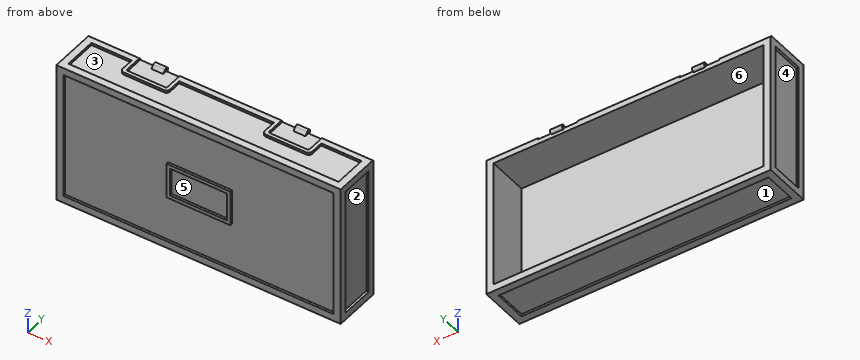
from build123d import *

# Parameters (mm, degrees)
SKETCH1_W                = 120
SKETCH1_H                = 60
BOSS_EXTRUDE1_DEPTH      = 20
SKETCH2_W                = 114
SKETCH2_H                = 54
CUT_EXTRUDE1_DEPTH       = 17
CUT_EXTRUDE2_DEPTH       = 1
CUT_EXTRUDE3_DEPTH       = 1
SKETCH5_W                = 54
SKETCH5_H                = 14
CUT_EXTRUDE4_DEPTH       = 1
SKETCH6_W                = 54
SKETCH6_H                = 14
CUT_EXTRUDE5_DEPTH       = 1
SKETCH7_W                = 114
SKETCH7_H                = 14
CUT_EXTRUDE6_DEPTH       = 1
SKETCH8_W                = 114
SKETCH8_H                = 54
CUT_EXTRUDE7_DEPTH       = 1
BOSS_EXTRUDE2_DEPTH      = 3
BOSS_EXTRUDE2_DEPTH_BACK = 0.5
CUT_EXTRUDE8_DEPTH       = 5
BOSS_EXTRUDE3_DEPTH      = 2
BOSS_EXTRUDE3_DEPTH_BACK = 0.5
CUT_EXTRUDE9_DEPTH       = 5
CUT_EXTRUDE10_DEPTH      = 23
CUT_EXTRUDE11_DEPTH      = 43
CUT_EXTRUDE12_DEPTH      = 43
BOSS_EXTRUDE5_DEPTH      = 1


with BuildPart() as part:
    # Sketch1 → Boss-Extrude1 (new body)
    with BuildSketch(Plane(origin=(0, 0, 0), x_dir=(1, 0, 0), z_dir=(0, 1, 0))):
        with Locations((60, 30)):
            Rectangle(SKETCH1_W, SKETCH1_H)
    extrude(amount=BOSS_EXTRUDE1_DEPTH)

    # Sketch2 → Cut-Extrude1 (cut)
    with BuildSketch(Plane(origin=(0, 20, 0), x_dir=(1, 0, 0), z_dir=(0, 1, 0))):
        with Locations((60, 30)):
            Rectangle(SKETCH2_W, SKETCH2_H)
    extrude(amount=-CUT_EXTRUDE1_DEPTH, mode=Mode.SUBTRACT)

    # Sketch3 → Cut-Extrude2 (cut)
    with BuildSketch(Plane.XY):
        with BuildLine():
            Line((38.5, 20), (21.5, 20))
            Line((21.5, 20), (21.5, 12))
            ThreePointArc((21.5, 12), (21.646446609, 11.646446609), (22, 11.5))
            Line((22, 11.5), (38, 11.5))
            ThreePointArc((38, 11.5), (38.353553391, 11.646446609), (38.5, 12))
            Line((38.5, 12), (38.5, 20))
        make_face()
        with BuildLine():
            Line((98.5, 12), (98.5, 20))
            Line((98.5, 20), (81.5, 20))
            Line((81.5, 20), (81.5, 12))
            ThreePointArc((81.5, 12), (81.646446609, 11.646446609), (82, 11.5))
            Line((82, 11.5), (98, 11.5))
            ThreePointArc((98, 11.5), (98.353553391, 11.646446609), (98.5, 12))
        make_face()
    extrude(amount=-CUT_EXTRUDE2_DEPTH, mode=Mode.SUBTRACT)

    # Sketch4 → Cut-Extrude3 (cut)
    with BuildSketch(Plane.XY):
        with BuildLine():
            Line((20, 17), (3, 17))
            Line((3, 17), (3, 3))
            Line((3, 3), (117, 3))
            Line((117, 3), (117, 17))
            Line((117, 17), (100, 17))
            Line((100, 17), (100, 11.5))
            ThreePointArc((100, 11.5), (99.560660172, 10.439339828), (98.5, 10))
            Line((98.5, 10), (81.5, 10))
            ThreePointArc((81.5, 10), (80.439339828, 10.439339828), (80, 11.5))
            Line((80, 11.5), (80, 17))
            Line((80, 17), (60, 17))
            Line((60, 17), (40, 17))
            Line((40, 17), (40, 11.5))
            ThreePointArc((40, 11.5), (39.560660172, 10.439339828), (38.5, 10))
            Line((38.5, 10), (21.5, 10))
            ThreePointArc((21.5, 10), (20.439339828, 10.439339828), (20, 11.5))
            Line((20, 11.5), (20, 17))
        make_face()
    extrude(amount=-CUT_EXTRUDE3_DEPTH, mode=Mode.SUBTRACT)

    # Sketch5 → Cut-Extrude4 (cut)
    with BuildSketch(Plane.ZY):
        with Locations((-30, 10)):
            Rectangle(SKETCH5_W, SKETCH5_H)
    extrude(amount=-CUT_EXTRUDE4_DEPTH, mode=Mode.SUBTRACT)

    # Sketch6 → Cut-Extrude5 (cut)
    with BuildSketch(Plane(origin=(120, 0, 0), x_dir=(0, 0, -1), z_dir=(1, 0, 0))):
        with Locations((30, 10)):
            Rectangle(SKETCH6_W, SKETCH6_H)
    extrude(amount=-CUT_EXTRUDE5_DEPTH, mode=Mode.SUBTRACT)

    # Sketch7 → Cut-Extrude6 (cut)
    with BuildSketch(Plane(origin=(0, 0, -60), x_dir=(-1, 0, 0), z_dir=(0, 0, -1))):
        with Locations((-60, 10)):
            Rectangle(SKETCH7_W, SKETCH7_H)
    extrude(amount=-CUT_EXTRUDE6_DEPTH, mode=Mode.SUBTRACT)

    # Sketch8 → Cut-Extrude7 (cut)
    with BuildSketch(Plane.XZ):
        with Locations((60, -30)):
            Rectangle(SKETCH8_W, SKETCH8_H)
    extrude(amount=-CUT_EXTRUDE7_DEPTH, mode=Mode.SUBTRACT)

    # Sketch9 → Boss-Extrude2 (add, two sides)
    with BuildSketch(Plane.XY.offset(-1)) as boss_extrude2_sk:
        Polygon((32.5, 20), (30, 20), (27.5, 20), (27.5, 18), (32.5, 18), align=None)
        Polygon((27.5, 20), (30, 20), (32.5, 20), (32.5, 21), (27.5, 21), align=None)
    extrude(amount=BOSS_EXTRUDE2_DEPTH)
    extrude(boss_extrude2_sk.sketch, amount=-BOSS_EXTRUDE2_DEPTH_BACK)

    # Sketch11 → Cut-Extrude8 (cut)
    with BuildSketch(Plane(origin=(32.5, 0, 0), x_dir=(0, 0, -1), z_dir=(1, 0, 0))):
        with BuildLine():
            Line((1, 18.085786438), (-0.207106781, 19.292893219))
            ThreePointArc((-0.207106781, 19.292893219), (-0.423879533, 20.382683432), (0.5, 21))
            Line((0.5, 21), (-2, 21))
            Line((-2, 21), (-2, 18))
            Line((-2, 18), (1, 18))
            Line((1, 18), (1, 18.085786438))
        make_face()
        with BuildLine():
            ThreePointArc((0.5, 21), (1.207106781, 20.707106781), (1.5, 20))
            Line((1.5, 20), (1.5, 21))
            Line((1.5, 21), (0.5, 21))
        make_face()
        with BuildLine():
            ThreePointArc((0.146446609, 19.646446609), (0.691341716, 19.538060234), (1, 20))
            Line((1, 20), (0.5, 20))
            Line((0.5, 20), (0.146446609, 19.646446609))
        make_face()
        with BuildLine():
            Line((0.5, 20), (1, 20))
            ThreePointArc((1, 20), (0.308658284, 20.461939766), (0.146446609, 19.646446609))
            Line((0.146446609, 19.646446609), (0.5, 20))
        make_face()
    extrude(amount=-CUT_EXTRUDE8_DEPTH, mode=Mode.SUBTRACT)

    # Sketch12 → Boss-Extrude3 (add, two sides)
    with BuildSketch(Plane.XY.offset(-1)) as boss_extrude3_sk:
        Polygon((87.5, 21), (87.5, 20), (87.5, 18), (92.5, 18), (92.5, 21), align=None)
    extrude(amount=BOSS_EXTRUDE3_DEPTH)
    extrude(boss_extrude3_sk.sketch, amount=-BOSS_EXTRUDE3_DEPTH_BACK)

    # Sketch13 → Cut-Extrude9 (cut)
    with BuildSketch(Plane(origin=(92.5, 0, 0), x_dir=(0, 0, -1), z_dir=(1, 0, 0))):
        with BuildLine():
            Line((1, 18.085786438), (-0.207106781, 19.292893219))
            ThreePointArc((-0.207106781, 19.292893219), (-0.423879533, 20.382683432), (0.5, 21))
            Line((0.5, 21), (-1, 21))
            Line((-1, 21), (-1, 18))
            Line((-1, 18), (1, 18))
            Line((1, 18), (1, 18.085786438))
        make_face()
        with BuildLine():
            ThreePointArc((0.146446609, 19.646446609), (0.691341716, 19.538060234), (1, 20))
            Line((1, 20), (0.5, 20))
            Line((0.5, 20), (0.146446609, 19.646446609))
        make_face()
        with BuildLine():
            Line((0.5, 20), (1, 20))
            ThreePointArc((1, 20), (0.308658284, 20.461939766), (0.146446609, 19.646446609))
            Line((0.146446609, 19.646446609), (0.5, 20))
        make_face()
        with BuildLine():
            ThreePointArc((0.5, 21), (1.207106781, 20.707106781), (1.5, 20))
            Line((1.5, 20), (1.5, 21))
            Line((1.5, 21), (0.5, 21))
        make_face()
    extrude(amount=-CUT_EXTRUDE9_DEPTH, mode=Mode.SUBTRACT)

    # Sketch14 → Cut-Extrude10 (cut)
    with BuildSketch(Plane.ZY):
        Polygon((0, 19.5), (0, 20), (-0.5, 20), align=None)
    extrude(amount=-CUT_EXTRUDE10_DEPTH, mode=Mode.SUBTRACT)

    # Sketch15 → Cut-Extrude11 (cut)
    with BuildSketch(Plane.ZY.offset(-38.5)):
        Polygon((0, 20), (-0.5, 20), (0, 19.5), align=None)
    extrude(amount=-CUT_EXTRUDE11_DEPTH, mode=Mode.SUBTRACT)

    # Sketch16 → Cut-Extrude12 (cut)
    with BuildSketch(Plane.ZY.offset(-98.5)):
        Polygon((0, 20), (-0.5, 20), (0, 19.5), align=None)
    extrude(amount=-CUT_EXTRUDE12_DEPTH, mode=Mode.SUBTRACT)

    # Sketch18 → Boss-Extrude5 (add)
    with BuildSketch(Plane(origin=(0, 0, 0), x_dir=(-1, 0, 0), z_dir=(0, -1, 0))):
        Polygon((-46.5, 36.75), (-48, 36), (-48, 24), (-60, 24), (-60, 22.5), (-46.5, 22.5), align=None)
        Polygon((-60, 24), (-72, 24), (-73.5, 23.25), (-73.5, 22.5), (-60, 22.5), align=None)
        Polygon((-72, 36), (-48, 36), (-46.5, 36.75), (-46.5, 37.5), (-73.5, 37.5), (-73.5, 23.25), (-72, 24), align=None)
    extrude(amount=-BOSS_EXTRUDE5_DEPTH)


solid = part.part
Input: part model. Units: mm. Frame: model coordinates. Face numbers are marked on the shaded views. A direction names the side the tool comes from. Give positions to 0.01 mm unless a question says otherwise; leave off trailing zeros. Loops run counter-clockwise (first coordinate to the right, second up) from the corner with the lowest first, then second, coordinate; pieces in that order, holes last. Notation, with made-up numbers: (27, -3.75) -> (84, -3.75) arc R23 cw to (84, 35.25) -> close; hole circle Ø4 at (76.5, 32.25). An arc over 180 degrees is marked (long way). Answer as a JSON object with one key per item and string values. Group by question number.
Item 1: Cut plane B-B, the plane x = 25. Return the cut outline in (y, z).
Item 2: Reachability of the marked faces 4, 5 and 6 from +Z, -Z, +X, -X, +Y, -Y: full face, straight path, thin tool, end or side. Return the list, or none.
Item 3: Pull-direction query (Z, two-part tool) for the marked faces 1, 2 and 3; classes: released by +Z, released by -Z, zero draft, split by the parting line, or undercut.
Item 4: Pin query (flat end, axial travel): P1, Ø0.8, axis at x = 119.5, y = 13, coming from the +Z side; P2, Ø3, axis at x = 79.5, z = -50, coming from the -Y side; P3, Ø5, axis at x = 87, y = 14, coming from the -Z side. Return the tip coordinate at first contact, or that it passes through.
Item 5: Cut plane A-A, the plane z = -50. Return the cut outline in (x, y), and give its area (3 significant figures).
Item 6: Cut plane C-C, the plane z = -28. Return the cut outline in (x, y), and give its area (3 significant figures).
Item 7: Line query: probe 1 along Z at (x, y) = (31, 4.25); probe 2 along Z at (x, y) = (51.5, 17.75); probe 3 along X at (y, z) = (9.75, -33). Output: solid intervals per line, ascending.
Checks:
{
 "1": {"outline": "(0, -60) -> (3, -60) -> (3, -59) -> (17, -59) -> (17, -60) -> (20, -60) -> (20, -57) -> (3, -57) -> (3, -3) -> (20, -3) -> (20, -1) -> (11.5, -1) -> (11.5, 0) -> (10, 0) -> (10, -1) -> (3, -1) -> (3, 0) -> (0, 0) -> (0, -3) -> (1, -3) -> (1, -57) -> (0, -57) -> close"},
 "2": {"face 4": "-X", "face 5": "-Y", "face 6": "+Y"},
 "3": {"face 1": "released by -Z", "face 2": "undercut", "face 3": "released by +Z"},
 "4": {"P1": "stops at z = 0", "P2": "stops at y = 1", "P3": "stops at z = -59"},
 "5": {"outline": "(0, 0) -> (3, 0) -> (3, 1) -> (117, 1) -> (117, 0) -> (120, 0) -> (120, 3) -> (119, 3) -> (119, 17) -> (120, 17) -> (120, 20) -> (117, 20) -> (117, 3) -> (3, 3) -> (3, 20) -> (0, 20) -> (0, 17) -> (1, 17) -> (1, 3) -> (0, 3) -> close", "area": "320 mm²"},
 "6": {"outline": "(0, 0) -> (3, 0) -> (3, 1) -> (46.5, 1) -> (46.5, 0) -> (48, 0) -> (48, 1) -> (72, 1) -> (72, 0) -> (73.5, 0) -> (73.5, 1) -> (117, 1) -> (117, 0) -> (120, 0) -> (120, 3) -> (119, 3) -> (119, 17) -> (120, 17) -> (120, 20) -> (117, 20) -> (117, 3) -> (3, 3) -> (3, 20) -> (0, 20) -> (0, 17) -> (1, 17) -> (1, 3) -> (0, 3) -> close", "area": "323 mm²"},
 "7": {"probe 1": "z = -59 to -57, -3 to -1", "probe 2": "z = -60 to -57, -3 to 0", "probe 3": "x = 1 to 3, 117 to 119"}
}
